from build123d import *

# Parameters (mm, degrees)
SKETCH1_W           = 304.8
SKETCH1_H           = 101.6
BOSS_EXTRUDE1_DEPTH = 254
SKETCH3_W           = 152.4
SKETCH3_H           = 101.6
CUT_EXTRUDE1_DEPTH  = 127
FILLET1_R           = 25.4
SKETCH4_R           = 25.4
BOSS_EXTRUDE2_DEPTH = 12.7


with BuildPart() as part:
    # Sketch1 → Boss-Extrude1 (new body)
    with BuildSketch(Plane.XY):
        with Locations((-152.4, 50.8)):
            Rectangle(SKETCH1_W, SKETCH1_H)
    extrude(amount=-BOSS_EXTRUDE1_DEPTH)

    # Sketch3 → Cut-Extrude1 (cut)
    with BuildSketch(Plane.XY):
        with Locations((-152.4, 50.8)):
            Rectangle(SKETCH3_W, SKETCH3_H)
    extrude(amount=-CUT_EXTRUDE1_DEPTH, mode=Mode.SUBTRACT)

    # Fillet1
    fillet1_edges = [part.edges().sort_by_distance(p)[0] for p in [
        (0, 50.8, -254),
        (0, 50.8, 0),
        (-304.8, 50.8, 0),
        (-304.8, 50.8, -254),
    ]]
    fillet(fillet1_edges, radius=FILLET1_R)

    # Sketch4 → Boss-Extrude2 (add)
    with BuildSketch(Plane(origin=(0, 101.6, 0), x_dir=(1, 0, 0), z_dir=(0, 1, 0))):
        with Locations(Location((-152.4, 190.5, 0), (0, 0, 270))):
            Circle(SKETCH4_R)
    extrude(amount=BOSS_EXTRUDE2_DEPTH)


solid = part.part
Model file for the job. Use its own axes, mm. A direction names the side the tool comes from. Give positions to 0.01 mm unless a question says otherwise; leave off trailing zeros. Write each loop counter-clockwise with the first axis right and the second up, starting at its lowest first coordinate (ties: lowest second). Pieces come first, ordered by that corner, then holes. Notation, with made-up numbers: (48, 57.5) -> (73, 57.5) arc R26 cw to (73, 74.5) -> close; hole circle Ø7 at (65, 0). An arc over 180 degrees is marked (long way). Write item = value, one per line.
(1) Flat gauge pins, fed straight in: P1, Ø5, axis at x = -53, z = -35, coming from the +Y side; P2, Ø4, axis at x = -252.5, z = -67, coming from the -Y side; P3, Ø4, axis at x = -190, y = 58.5, coming from the +Z side. Where does each tip first touch, or does it go through?
Determined:
P1 = 101.6
P2 = 0
P3 = -127
(2) Probe line 1 along X through (y, z) = (81.5, -105.5); line 2 along Y through (x, z) = (-66.5, -172); line 3 along Z through (x, y) = (-103, 36). List the from-to ranges inside material, lowest first.
Determined:
line_1 = -304.8 to -228.6, -76.2 to 0
line_2 = 0 to 101.6
line_3 = -254 to -127
(3) Tool access for faces 5 (the face through (-51, 52, 0)), 6 (the face through (-76.2, 50, -63)), 7 (the face through (-151.283, 107.861, -215.875)): list every direction of +Z, -Z, +X, -X, +Y, -Y with a clear straight run to the whole face (end or side of a thin tool).
Determined:
face_5 = +Z, +X, -X, +Y, -Y
face_6 = +Z, +Y, -Y
face_7 = +Y
(4) Slice it at C-C, the plane y = 23. Give the cut face in (x, z), then the cut area to 3 significant figures.
Determined:
outline = (-304.8, -228.6) arc R25.4 ccw to (-279.4, -254) -> (-25.4, -254) arc R25.4 ccw to (0, -228.6) -> (0, -25.4) arc R25.4 ccw to (-25.4, 0) -> (-76.2, 0) -> (-76.2, -127) -> (-228.6, -127) -> (-228.6, 0) -> (-279.4, 0) arc R25.4 ccw to (-304.8, -25.4) -> close
area = 57,500 mm2
(5) Slice it at D-D, the plane z = -190.5. Give the cut face in (x, y), then the cut area to 3 significant figures.
Determined:
outline = (-304.8, 0) -> (0, 0) -> (0, 101.6) -> (-127, 101.6) -> (-127, 114.3) -> (-177.8, 114.3) -> (-177.8, 101.6) -> (-304.8, 101.6) -> close
area = 31,600 mm2
(6) Slice it at A-A, the plane z = -117.5. Give the cut face in (x, y), then the cut area to 3 significant figures.
Determined:
outline = (-304.8, 0) -> (-228.6, 0) -> (-228.6, 101.6) -> (-304.8, 101.6) -> close; (-76.2, 0) -> (0, 0) -> (0, 101.6) -> (-76.2, 101.6) -> close
area = 15,500 mm2
(7) Mould opens along X. For faces 1 (the face through (0, 50, -126)), 2 (the face through (-228.6, 50, -63)), 3 (the face through (-155, 101.6, -153)), 4 (the face through (-304.8, 50, -126)) say: released by +X, released by -X, zero draft, split by the parting line, or undercut.
Determined:
face_1 = released by +X
face_2 = undercut
face_3 = zero draft
face_4 = released by -X
(8) Slice it at B-B, the plane x = -152.4. Give the cut face in (y, z), then the cut area to 3 significant figures.
Determined:
outline = (0, -254) -> (101.6, -254) -> (101.6, -215.9) -> (114.3, -215.9) -> (114.3, -165.1) -> (101.6, -165.1) -> (101.6, -127) -> (0, -127) -> close
area = 13,500 mm2
